from build123d import *

# Parameters (mm, degrees)
ESQUISSE1_R              = 11
BOSS_EXTRU_1_DEPTH       = 7.5
ESQUISSE3_R              = 15
BOSS_EXTRU_2_DEPTH       = 6.5
CHANFREIN1_SIZE          = 0.5
CHANFREIN2_SIZE          = 1
ESQUISSE4_R              = 14.5
ENL_V_MAT_EXTRU_1_DEPTH  = 3.5
ESQUISSE5_R              = 4.5
ENL_V_MAT_EXTRU_2_DEPTH  = 1.5
ESQUISSE6_R              = 7
ENL_V_MAT_EXTRU_3_DEPTH  = 1
ESQUISSE20_R             = 8
ENL_V_MAT_EXTRU_4_DEPTH  = 8
F_2_0_2_DIAMETER_HOLE1_D = 2


with BuildPart() as part:
    # Esquisse1 → Boss.-Extru.1 (new body)
    with BuildSketch(Plane(origin=(0, 0, 0), x_dir=(1, 0, 0), z_dir=(0, 1, 0))):
        with Locations(Location((0, 0, 0), (0, 0, 270))):
            Circle(ESQUISSE1_R)
    extrude(amount=BOSS_EXTRU_1_DEPTH)

    # Esquisse3 → Boss.-Extru.2 (add)
    with BuildSketch(Plane(origin=(0, 7.5, 0), x_dir=(1, 0, 0), z_dir=(0, 1, 0))):
        with Locations(Location((0, 0, 0), (0, 0, 90))):
            Circle(ESQUISSE3_R)
    extrude(amount=BOSS_EXTRU_2_DEPTH)

    # Chanfrein1
    chanfrein1_edges = [part.edges().sort_by_distance(p)[0] for p in [
        (0, 0, -11),
    ]]
    chamfer(chanfrein1_edges, length=CHANFREIN1_SIZE)

    # Chanfrein2
    chanfrein2_edges = [part.edges().sort_by_distance(p)[0] for p in [
        (0, 7.5, -11),
    ]]
    chamfer(chanfrein2_edges, length=CHANFREIN2_SIZE)

    # Esquisse4 → Enlèv. mat.-Extru.1 (cut)
    with BuildSketch(Plane(origin=(0, 14, 0), x_dir=(1, 0, 0), z_dir=(0, 1, 0))):
        with Locations(Location((0, 0, 0), (0, 0, 270))):
            Circle(ESQUISSE4_R)
    extrude(amount=-ENL_V_MAT_EXTRU_1_DEPTH, mode=Mode.SUBTRACT)

    # Esquisse5 → Enlèv. mat.-Extru.2 (cut)
    with BuildSketch(Plane(origin=(0, 10.5, 0), x_dir=(1, 0, 0), z_dir=(0, 1, 0))):
        with Locations(Location((0, 0, 0), (0, 0, 270))):
            Circle(ESQUISSE5_R)
    extrude(amount=-ENL_V_MAT_EXTRU_2_DEPTH, mode=Mode.SUBTRACT)

    # Esquisse6 → Enlèv. mat.-Extru.3 (cut)
    with BuildSketch(Plane(origin=(0, 9, 0), x_dir=(1, 0, 0), z_dir=(0, 1, 0))):
        with Locations(Location((0, 0, 0), (0, 0, 270))):
            Circle(ESQUISSE6_R)
    extrude(amount=-ENL_V_MAT_EXTRU_3_DEPTH, mode=Mode.SUBTRACT)

    # Esquisse20 → Enlèv. mat.-Extru.4 (cut)
    with BuildSketch(Plane(origin=(0, 8, 0), x_dir=(1, 0, 0), z_dir=(0, 1, 0))):
        with Locations(Location((0, 0, 0), (0, 0, 270))):
            Circle(ESQUISSE20_R)
    extrude(amount=-ENL_V_MAT_EXTRU_4_DEPTH, mode=Mode.SUBTRACT)

    # Ø2.0 (2) Diameter Hole1 (through all)
    with Locations(Plane(origin=(0, 7.5, 0), x_dir=(-1, 0, 0), z_dir=(0, -1, 0))):
        with Locations((-9.5, 8.9)):
            Hole(F_2_0_2_DIAMETER_HOLE1_D / 2)


solid = part.part
Could you check a few things on this model? Use its own coordinates, in mm. A direction names the side the tool comes from. Round coordinates to 2 decimals unless told otherwise and drop trailing zeros. Write each loop counter-clockwise with the first axis right and the second up, starting at its lowest first coordinate (ties: lowest second). Pieces come first, ordered by that corner, then holes. Notation, with made-up numbers: (-10, -36.75) - (27, -36.75) arc R23 ccw to (27, -10.75) - close; hole circle Ø8 at (25.5, 18.25). An arc over 180 degrees is marked (long way). Put each result on its own line as item: value. Start each with the question number.
(1) I want a section at B-B, the plane z = 0. Please give me the cut outline in (x, y), plus the area to 3 significant figures.
(2) I want a section at C-C, the plane y = 11. Please give me the cut outline in (x, z), plus the area to 3 significant figures.
(3) I need wall thicknesses on probe 1 along X at (y, z) = (9.5, 0); probe 2 along Y at (x, z) = (3, 7.5); probe 3 along Y at (x, z) = (-12, -1.5). Which ranges of each line are inside material? Lowest first, please.
(4) I want a section at A-A, the plane x = 0. Please give me the cut outline in (y, z).
(5) Thinking about a two-plate mould opening in Z: for faces 1 (the flat face through (-10, 7.5, 7)), 2 (the cylindrical face through (-7.81, 4.06, -1.73)), 3 (the cylindrical face through (-0.66, 10.704, 14.985)), which applies, released by +Z, released by -Z, zero draft, split by the parting line, or undercut?
(6) Will these pins go through, and if not, where does the flat tip stop? pin 1 (14.5 mm diameter, centred on x = 0, z = 0, fed in from +Y); pin 2 (1 mm diameter, centred on y = 12.5, z = 6.5, fed in from -X); pin 3 (5 mm diameter, centred on y = 10.5, z = 8, fed in from -X).
(7) I want a section at D-D, the plane y = 3.5. Please give me the cut outline in (x, z).
(8) For faces 4 (the cylindrical face through (-6.834, 8.507, -1.517)), 5 (the cylindrical face through (-5.554, 12.274, 13.394)), 6 (the cylindrical face through (8.7, 9, -8.3)), which set-ups out of +Z, -Z, +X, -X, +Y, -Y let a thin tool reach every point of the face, with its end or its side?
Here are the results:
1. outline: (-15, 7.5) - (-12, 7.5) - (-11, 6.5) - (-11, 0.5) - (-10.5, 0) - (-8, 0) - (-8, 8) - (-7, 8) - (-7, 9) - (-4.5, 9) - (-4.5, 10.5) - (-14.5, 10.5) - (-14.5, 14) - (-15, 14) - close; (4.5, 9) - (7, 9) - (7, 8) - (8, 8) - (8, 0) - (10.5, 0) - (11, 0.5) - (11, 6.5) - (12, 7.5) - (15, 7.5) - (15, 14) - (14.5, 14) - (14.5, 10.5) - (4.5, 10.5) - close
1. area: 104 mm^2
2. outline: circle Ø30 at (0, 0); hole circle Ø29 at (0, 0)
2. area: 46.3 mm^2
3. probe 1: x = -15 to -4.5, 4.5 to 15
3. probe 2: y = 0 to 10.5
3. probe 3: y = 7.5 to 10.5
4. outline: (0, -10.5) - (0.5, -11) - (6.5, -11) - (7.5, -12) - (7.5, -15) - (14, -15) - (14, -14.5) - (10.5, -14.5) - (10.5, -4.5) - (9, -4.5) - (9, -7) - (8, -7) - (8, -8) - (0, -8) - close; (0, 8) - (8, 8) - (8, 7) - (9, 7) - (9, 4.5) - (10.5, 4.5) - (10.5, 14.5) - (14, 14.5) - (14, 15) - (7.5, 15) - (7.5, 12) - (6.5, 11) - (0.5, 11) - (0, 10.5) - close
5. face 1: zero draft
5. face 2: undercut
5. face 3: split by the parting line
6. pin 1: stops at y = 10.5
6. pin 2: stops at x = -13.75
6. pin 3: stops at x = -13.96
7. outline: circle Ø22 at (0, 0); hole circle Ø16 at (0, 0)
8. face 4: -Y
8. face 5: +Y
8. face 6: +Y, -Y
